Could you check a few things on this drawing? It's one solid part, dimensions in mm from its lowest x, y, z. A direction names the side the tool comes from. Coordinates: 2 decimals unless noted, no trailing zeros. Order: outer loops, then holes, each group sorted by start corner. A loop starts at its lowest first (then second) coordinate and runs counter-clockwise, first axis right, second up. Notation, with made-up numbers: M -1.5,-11 L 52.5,-11 A23 ccw 52.5,8 Z; hole C 81,80.25 d8. An arc over 180 degrees is marked long. One line per question, with ' | ' between items. Start each with the question number.
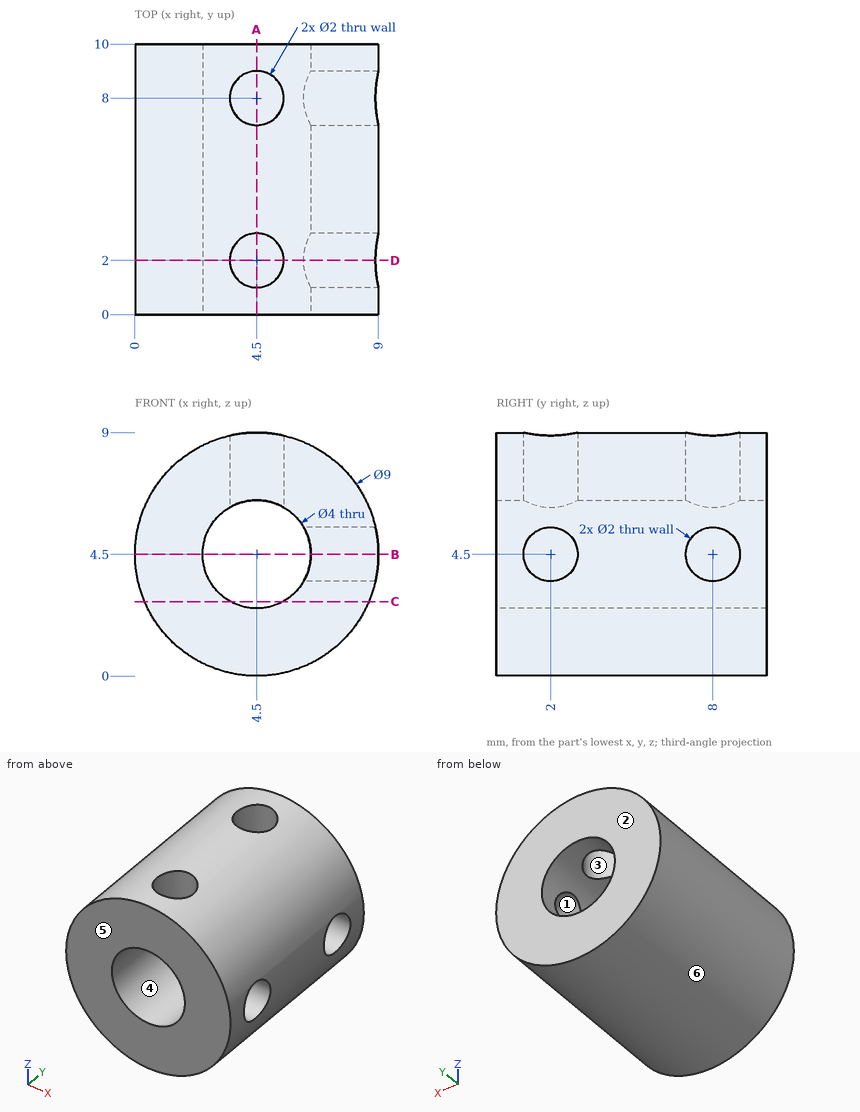
1. Which directions (+Z, -Z, +X, -X, +Y, -Y) give clear straight access to the entire face, cutting with the end or side of a thin tool? Please do the marked faces 1, 2 and 3.
2. Imagine slicing it at A-A (x = 4.5). List the corners of the cut face in (y, z) for me, then the cut area to 3 significant figures.
3. Will these pins go through, and if not, where does the flat tip stop? pin 1 (1 mm diameter, centred on y = 5.5, z = 6.5, fed in from -X); pin 2 (1.5 mm diameter, centred on x = 6.5, y = 3.5, fed in from -Z); pin 3 (1 mm diameter, centred on x = 3.5, y = 8.5, fed in from +Z).
4. I need wall thicknesses on line 1 (X direction, y = 6, z = 4.5); line 2 (Y direction, x = 7.5, z = 5); line 3 (X direction, y = 3.5, z = 3.75). Which ranges of each line are inside material? Lowest first, please.
5. Imagine slicing it at B-B (z = 4.5). List the corners of the cut face in (x, y) for me, then the cut area to 3 significant figures.
6. We'd pull the mould along Z, two halves only. Please class the marked faces 4, 5 and 6: released by +Z, released by -Z, zero draft, split by the parting line, or undercut.
7. Imagine slicing it at D-D (y = 2). List the corners of the cut face in (x, z) for me, then the cut area to 3 significant figures.
8. Imagine slicing it at C-C (z = 2.75). List the corners of the cut face in (x, y) for me, then the cut area to 3 significant figures.
Entries:
1) face 1: +X | face 2: +Z, -Z, +X, -X, +Y | face 3: +Z
2) outline: M 0,0 L 10,0 L 10,2.5 L 0,2.5 Z; M 0,6.5 L 1,6.5 L 1,9 L 0,9 Z; M 3,6.5 L 7,6.5 L 7,9 L 3,9 Z; M 9,6.5 L 10,6.5 L 10,9 L 9,9 Z | area: 40.0 mm²
3) pin 1: x = 0.26 | pin 2: z = 0.18 | pin 3: z = 8.96
4) line 1: 0 to 2.5, 6.5 to 9 | line 2: 0 to 1.13, 2.87 to 7.13, 8.87 to 10 | line 3: 0.06 to 2.65, 6.35 to 8.94
5) outline: M 0,0 L 2.5,0 L 2.5,10 L 0,10 Z; M 6.5,0 L 9,0 L 9,1 L 6.5,1 Z; M 6.5,3 L 9,3 L 9,7 L 6.5,7 Z; M 6.5,9 L 9,9 L 9,10 L 6.5,10 Z | area: 40.0 mm²
6) face 4: undercut | face 5: zero draft | face 6: split by the parting line
7) outline: M 3.5,6.23 L 3.5,8.89 A4.5 ccw long 8.89,3.5 L 6.23,3.5 A2 cw long Z; M 5.5,6.23 A2 cw 6.23,5.5 L 8.89,5.5 A4.5 ccw 5.5,8.89 Z | area: 40.9 mm²
8) outline: M 0.35,0 L 3.53,0 L 3.53,10 L 0.35,10 Z; M 5.47,0 L 8.65,0 L 8.65,10 L 5.47,10 Z | area: 63.6 mm²
